Drawing for the job (mm, zero at the part's lowest x, y, z). A direction names the side the tool comes from. Give positions to 0.01 mm unless a question says otherwise; leave off trailing zeros. Write each loop counter-clockwise with the first axis right and the second up, starting at its lowest first coordinate (ties: lowest second). Pieces come first, ordered by that corner, then holes. Notation, with made-up numbers: M 47,12 L 97,12 A14 cw 97,33 Z; hole C 79.5,62.5 d4. An arc over 180 degrees is marked long. Use CSV: the item, a comma, the result in double quotes. Start each with the question number.
1. Band-saw the part on C-C, the plane y = 15.75. List the corners of the cut face in (x, z).
2. Band-saw the part on D-D, the plane x = 2.5. List the corners of the cut face in (y, z).
3. Drill centre lines: line 1 along X through (y, z) = (10, 14.5); line 2 along Y through (x, z) = (13.5, 7.5); line 3 along Z through (x, y) = (2, 18.5). Where is each one in solid material? Low to high. Write a range as from..to.
4. Drop flat-ended pins along their axis: pin 1 Ø2.5 at (y, z) = (17, 2) entering from -X; pin 2 Ø0.9 at (x, y) = (1.5, 26) entering from +Z; pin 3 Ø10 at (x, z) = (9, 19.5) entering from +Y; pin 4 Ø1.5 at (x, z) = (1, 26) entering from +Y. Give the stop position or say it passes through.
5. 3-axis set-ups, long thin cutter, end or side, ignore diameter. For the marked faces 1, 2 and 3: which of +Z, -Z, +X, -X, +Y, -Y reach the whole face in a straight line?
6. Band-saw the part on A-A, the plane z = 14.75. List the corners of the cut face in (x, y).
7. Band-saw the part on B-B, the plane x = 10. List the corners of the cut face in (y, z).
8. Mould opens along X. For the marked faces 4, 5, 6 and 7 say: pulls with the +X half, pulls with the -X half, needs draft (parallel to the pull), parting line crosses it, or undercut.
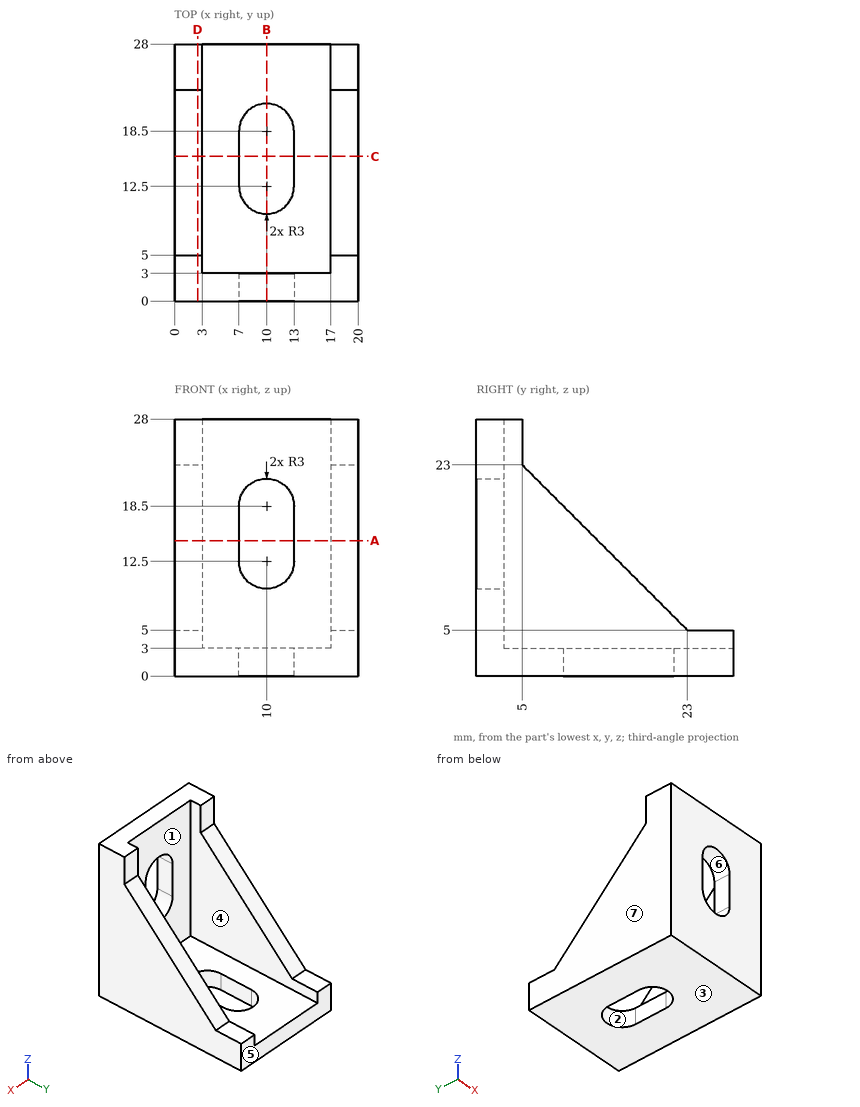
Output:
1,outline,"M 0,0 L 7,0 L 7,3 L 3,3 L 3,12.25 L 0,12.25 Z; M 13,0 L 20,0 L 20,12.25 L 17,12.25 L 17,3 L 13,3 Z"
2,outline,"M 0,0 L 28,0 L 28,5 L 23,5 L 5,23 L 5,28 L 0,28 Z"
3,line 1,"x = 0..3, 17..20"
3,line 2,"y = 0..3"
3,line 3,"z = 0..9.5"
4,pin 1,"stops at x = 0"
4,pin 2,"stops at z = 5"
4,pin 3,"stops at y = 3"
4,pin 4,"stops at y = 5"
5,face 1,"+Z, +Y"
5,face 2,"+Z, -Z"
5,face 3,"-Z, +X, -X, +Y, -Y"
6,outline,"M 0,0 L 7,0 L 7,3 L 3,3 L 3,13.25 L 0,13.25 Z; M 13,0 L 20,0 L 20,13.25 L 17,13.25 L 17,3 L 13,3 Z"
7,outline,"M 0,0 L 9.5,0 L 9.5,3 L 3,3 L 3,9.5 L 0,9.5 Z; M 0,21.5 L 3,21.5 L 3,28 L 0,28 Z; M 21.5,0 L 28,0 L 28,3 L 21.5,3 Z"
8,face 4,"undercut"
8,face 5,"needs draft"
8,face 6,"undercut"
8,face 7,"pulls with the -X half"
